from build123d import *

# Parameters (mm, degrees)
SKETCH1_W           = 10
SKETCH1_H           = 22
BOSS_EXTRUDE1_DEPTH = 42
SKETCH2_W           = 4.5
SKETCH2_H           = 16
CUT_EXTRUDE1_DEPTH  = 36
SKETCH4_W           = 2.4
SKETCH4_H           = 18.2
CUT_EXTRUDE3_DEPTH  = 37
SKETCH5_W           = 4
SKETCH5_H           = 15
CUT_EXTRUDE4_DEPTH  = 19
SKETCH6_W           = 1.2
SKETCH6_H           = 16.5
CUT_EXTRUDE5_DEPTH  = 20.5
SKETCH8_W           = 3
SKETCH8_H           = 14.5
CUT_EXTRUDE6_DEPTH  = 15.5
SKETCH9_W           = 1.2
SKETCH9_H           = 16.5
CUT_EXTRUDE7_DEPTH  = 16.5
SKETCH10_W          = 12
SKETCH10_H          = 16
CUT_EXTRUDE8_DEPTH  = 2.5
SKETCH12_W          = 9
SKETCH12_H          = 2.9
SKETCH12_W_2        = 7.5
SKETCH12_H_2        = 2.75
CUT_EXTRUDE11_DEPTH = 10
CUT_EXTRUDE12_REACH = 12
SKETCH13_W          = 9
SKETCH13_H          = 0.6
SKETCH13_W_2        = 7.5
SKETCH13_H_2        = 0.25
CUT_EXTRUDE13_REACH = 12
SKETCH14_W          = 9
SKETCH14_H          = 0.1
SKETCH14_W_2        = 6.5
SKETCH14_H_2        = 0.25
SKETCH15_W          = 2
SKETCH15_H          = 10
SKETCH15_W_2        = 11
CUT_EXTRUDE14_DEPTH = 7
SKETCH16_W          = 2
SKETCH16_H          = 10
SKETCH16_W_2        = 7
CUT_EXTRUDE15_DEPTH = 10
SKETCH17_W          = 3
SKETCH17_H          = 10
CUT_EXTRUDE16_DEPTH = 10
SKETCH18_W          = 10
SKETCH18_H          = 52
BOSS_EXTRUDE3_DEPTH = 30
SKETCH21_W          = 1.3
SKETCH21_H          = 6
CUT_EXTRUDE18_DEPTH = 28
FILLET1_R           = 2
FILLET3_R           = 1
CUT_EXTRUDE19_DEPTH = 28
FILLET4_R           = 2


with BuildPart() as part:
    # Sketch1 → Boss-Extrude1 (new body)
    with BuildSketch(Plane.XY):
        Rectangle(SKETCH1_W, SKETCH1_H)
    extrude(amount=BOSS_EXTRUDE1_DEPTH)

    # Sketch2 → Cut-Extrude1 (cut)
    with BuildSketch(Plane.XY.offset(42)):
        with Locations((2.75, 0)):
            Rectangle(SKETCH2_W, SKETCH2_H)
    extrude(amount=-CUT_EXTRUDE1_DEPTH, mode=Mode.SUBTRACT)

    # Sketch4 → Cut-Extrude3 (cut)
    with BuildSketch(Plane.XY.offset(42)):
        with Locations((2.2, 0.373327294)):
            Rectangle(SKETCH4_W, SKETCH4_H)
    extrude(amount=-CUT_EXTRUDE3_DEPTH, mode=Mode.SUBTRACT)

    # Sketch5 → Cut-Extrude4 (cut)
    with BuildSketch(Plane.XY.offset(42)):
        with Locations((-3, 0)):
            Rectangle(SKETCH5_W, SKETCH5_H)
    extrude(amount=-CUT_EXTRUDE4_DEPTH, mode=Mode.SUBTRACT)

    # Sketch6 → Cut-Extrude5 (cut)
    with BuildSketch(Plane.XY.offset(42)):
        with Locations((-2.4, 0)):
            Rectangle(SKETCH6_W, SKETCH6_H)
    extrude(amount=-CUT_EXTRUDE5_DEPTH, mode=Mode.SUBTRACT)

    # Sketch8 → Cut-Extrude6 (cut)
    with BuildSketch(Plane(origin=(0, 0, 0), x_dir=(-1, 0, 0), z_dir=(0, 0, -1))):
        with Locations((3.5, 0)):
            Rectangle(SKETCH8_W, SKETCH8_H)
    extrude(amount=-CUT_EXTRUDE6_DEPTH, mode=Mode.SUBTRACT)

    # Sketch9 → Cut-Extrude7 (cut)
    with BuildSketch(Plane(origin=(0, 0, 0), x_dir=(-1, 0, 0), z_dir=(0, 0, -1))):
        with Locations((3.1, 0)):
            Rectangle(SKETCH9_W, SKETCH9_H)
    extrude(amount=-CUT_EXTRUDE7_DEPTH, mode=Mode.SUBTRACT)

    # Sketch10 → Cut-Extrude8 (cut)
    with BuildSketch(Plane.ZY.offset(5)):
        with Locations((8, 0)):
            Rectangle(SKETCH10_W, SKETCH10_H)
    extrude(amount=-CUT_EXTRUDE8_DEPTH, mode=Mode.SUBTRACT)

    # Sketch12 → Cut-Extrude11 (cut)
    with BuildSketch(Plane.ZY.offset(5)):
        with Locations((32.5, -9.55)):
            Rectangle(SKETCH12_W, SKETCH12_H)
        with Locations((8.75, -9.625)):
            Rectangle(SKETCH12_W_2, SKETCH12_H_2)
    extrude(amount=-CUT_EXTRUDE11_DEPTH, mode=Mode.SUBTRACT)

    # Sketch13 → Cut-Extrude12 (cut, up to next)
    with BuildSketch(Plane.ZY.offset(5), mode=Mode.PRIVATE) as cut_extrude12_sk1:
        with Locations((32.5, -7.8)):
            Rectangle(SKETCH13_W, SKETCH13_H)
    cut_extrude12_tool1 = extrude(cut_extrude12_sk1.sketch, amount=-CUT_EXTRUDE12_REACH, mode=Mode.PRIVATE) & part.part
    add(cut_extrude12_tool1.solids().sort_by_distance((-5, -7.8, 32.5))[0], mode=Mode.SUBTRACT)
    # Sketch13 → Cut-Extrude12 (cut, up to next)
    with BuildSketch(Plane.ZY.offset(5), mode=Mode.PRIVATE) as cut_extrude12_sk2:
        with Locations((8.75, -8.125)):
            Rectangle(SKETCH13_W_2, SKETCH13_H_2)
    cut_extrude12_tool2 = extrude(cut_extrude12_sk2.sketch, amount=-CUT_EXTRUDE12_REACH, mode=Mode.PRIVATE) & part.part
    add(cut_extrude12_tool2.solids().sort_by_distance((-5, -8.125, 8.75))[0], mode=Mode.SUBTRACT)

    # Sketch14 → Cut-Extrude13 (cut, up to next)
    with BuildSketch(Plane(origin=(5, 0, 0), x_dir=(0, 0, -1), z_dir=(1, 0, 0)), mode=Mode.PRIVATE) as cut_extrude13_sk1:
        with Locations((-32.5, -8.05)):
            Rectangle(SKETCH14_W, SKETCH14_H)
    cut_extrude13_tool1 = extrude(cut_extrude13_sk1.sketch, amount=-CUT_EXTRUDE13_REACH, mode=Mode.PRIVATE) & part.part
    add(cut_extrude13_tool1.solids().sort_by_distance((5, -8.05, 32.5))[0], mode=Mode.SUBTRACT)
    # Sketch14 → Cut-Extrude13 (cut, up to next)
    with BuildSketch(Plane(origin=(5, 0, 0), x_dir=(0, 0, -1), z_dir=(1, 0, 0)), mode=Mode.PRIVATE) as cut_extrude13_sk2:
        with Locations((-9.25, -8.125)):
            Rectangle(SKETCH14_W_2, SKETCH14_H_2)
    cut_extrude13_tool2 = extrude(cut_extrude13_sk2.sketch, amount=-CUT_EXTRUDE13_REACH, mode=Mode.PRIVATE) & part.part
    add(cut_extrude13_tool2.solids().sort_by_distance((5, -8.125, 9.25))[0], mode=Mode.SUBTRACT)

    # Sketch15 → Cut-Extrude14 (cut, through all)
    with BuildSketch(Plane.ZY.offset(1)):
        with Locations((41, 0)):
            Rectangle(SKETCH15_W, SKETCH15_H)
        with Locations((31.5, 0)):
            Rectangle(SKETCH15_W_2, SKETCH15_H)
    extrude(amount=-CUT_EXTRUDE14_DEPTH, mode=Mode.SUBTRACT)

    # Sketch16 → Cut-Extrude15 (cut)
    with BuildSketch(Plane.ZY.offset(2)):
        with Locations((1, 0)):
            Rectangle(SKETCH16_W, SKETCH16_H)
        with Locations((8.5, 0)):
            Rectangle(SKETCH16_W_2, SKETCH16_H)
    extrude(amount=-CUT_EXTRUDE15_DEPTH, mode=Mode.SUBTRACT)

    # Sketch17 → Cut-Extrude16 (cut)
    with BuildSketch(Plane(origin=(0, 0, 2), x_dir=(-1, 0, 0), z_dir=(0, 0, -1))):
        with Locations((-3.5, 0)):
            Rectangle(SKETCH17_W, SKETCH17_H)
    extrude(amount=-CUT_EXTRUDE16_DEPTH, mode=Mode.SUBTRACT)

    # Sketch18 → Boss-Extrude3 (add)
    with BuildSketch(Plane(origin=(0, 11, 0), x_dir=(1, 0, 0), z_dir=(0, 1, 0))):
        with Locations((0, -21)):
            Rectangle(SKETCH18_W, SKETCH18_H)
    extrude(amount=BOSS_EXTRUDE3_DEPTH)

    # Sketch21 → Cut-Extrude18 (cut)
    with BuildSketch(Plane.XZ.offset(-8)):
        with Locations((-4.35, 9)):
            Rectangle(SKETCH21_W, SKETCH21_H)
    extrude(amount=-CUT_EXTRUDE18_DEPTH, mode=Mode.SUBTRACT)

    # Fillet1
    fillet1_edges = [part.edges().sort_by_distance(p)[0] for p in [
        (5, 26, -5),
        (-5, 26, -5),
        (5, 26, 47),
        (-5, 26, 47),
    ]]
    fillet(fillet1_edges, radius=FILLET1_R)

    # Fillet3
    fillet3_edges = [part.edges().sort_by_distance(p)[0] for p in [
        (-3.7, 8.25, 9),
    ]]
    fillet(fillet3_edges, radius=FILLET3_R)

    # Sketch22 → Cut-Extrude19 (cut)
    with BuildSketch(Plane(origin=(0, 41, 0), x_dir=(1, 0, 0), z_dir=(0, 1, 0))):
        with BuildLine():
            Line((-5, -41.5), (-5, -0.5))
            ThreePointArc((-5, -0.5), (-1, 3.5), (3, -0.5))
            Line((3, -0.5), (3, -41.5))
            ThreePointArc((3, -41.5), (-1, -45.5), (-5, -41.5))
        make_face()
    extrude(amount=-CUT_EXTRUDE19_DEPTH, mode=Mode.SUBTRACT)

    # Fillet4
    fillet4_edges = [part.edges().sort_by_distance(p)[0] for p in [
        (-3.7, 13, 9),
    ]]
    fillet(fillet4_edges, radius=FILLET4_R)


solid = part.part
Verification items for the finished model (mm, model axes). A direction names the side the tool comes from. Coordinates: 2 decimals unless noted, no trailing zeros. Order: outer loops, then holes, each group sorted by start corner. A loop starts at its lowest first (then second) coordinate and runs counter-clockwise, first axis right, second up. Notation, with made-up numbers: M -17.5,-39.75 L -8.5,-39.75 A18 ccw -8.5,-30.75 Z; hole C -32,-5 d2. An arc over 180 degrees is marked long. Write each question's results on one line, items separated by ' | '.
1) Section check B-B on z = 18.5. Record the cut outline in (x, y), plus the area to 3 significant figures.
Solved:
outline: M -5,-11 L 5,-11 L 5,-8 L 3.4,-8 L 3.4,-8.73 L 1,-8.73 L 1,-8 L 0.5,-8 L 0.5,8 L 1,8 L 1,9.47 L 3.4,9.47 L 3.4,8 L 5,8 L 5,41 L 3,41 L 3,13 L -5,13 Z | area: 219 mm²
2) Release check for a two-part mould opening along Y. For faces 1 (the face through (5, -10, 20)), 2 (the face through (0, -11, 39)), 3 (the face through (-4, 8, 4)) record: pulls with the +Y half, pulls with the -Y half, needs draft (parallel to the pull), parting line crosses it, or undercut.
Solved:
face 1: needs draft | face 2: pulls with the -Y half | face 3: undercut
3) Section check C-C on y = 35.5. Record the cut outline in (x, z), plus the area to 3 significant figures.
Solved:
outline: M -5,-3 A2 ccw -3,-5 L 3,-5 A2 ccw 5,-3 L 5,45 A2 ccw 3,47 L -3,47 A2 ccw -5,45 L -5,41.5 A4 cw 3,41.5 L 3,0.5 A4 cw -5,0.5 Z | area: 138 mm²
4) Gauge pin test, flat ends, axial feed: pin 1 Ø3 at (x, y) = (0, 6.5) entering from +Z; pin 2 Ø5 at (x, z) = (-2.5, 17.5) entering from +Y; pin 3 Ø8 at (y, z) = (2, 23) entering from +X. Record the tip position at first contact, or that the pin passes through.
Solved:
pin 1: stops at z = 42 | pin 2: stops at y = 13 | pin 3: stops at x = 0.5
5) Scan lines: line 1 along Z through (x, y) = (0, -2); line 2 along Y through (x, z) = (-1.5, 35.5); line 3 along Y through (x, z) = (2.25, 20). Record each from-to range of solid material in increasing order. Write a range as [from, to].
Solved:
line 1: z = [2, 5], [12, 26], [37, 40] | line 2: y = [-8.1, -7.5], [7.5, 13] | line 3: y = [-11, -8.73], [9.47, 13]
6) Section check A-A on y = 0. Record the cut outline in (x, z).
Solved:
outline: M -5,15.5 L -3.7,15.5 L -3.7,16.5 L -2.5,16.5 L -2.5,15.5 L -2,15.5 L -2,12 L 0.5,12 L 0.5,26 L -1,26 L -1,23 L -1.8,23 L -1.8,21.5 L -3,21.5 L -3,23 L -5,23 Z; M -2,2 L 2,2 L 2,5 L -2,5 Z; M -1,37 L 0.5,37 L 0.5,40 L -1,40 Z
7) Access from +Z, -Z, +X, -X, +Y, -Y to the whole of each face (thin tool, end or side, straight path). Record for faces 4 (the face through (4, 8, 24)), 5 (the face through (-0.9, 27.2, 45.5)), 6 (the face through (4, 7, 6)), 7 (the face through (0, 0, 26)), 8 (the face through (0, 11, -3)).
Solved:
face 4: +Z, +X | face 5: +Y | face 6: +Z, +X, -Y | face 7: +X, -X | face 8: -Z, +X, -X, -Y
